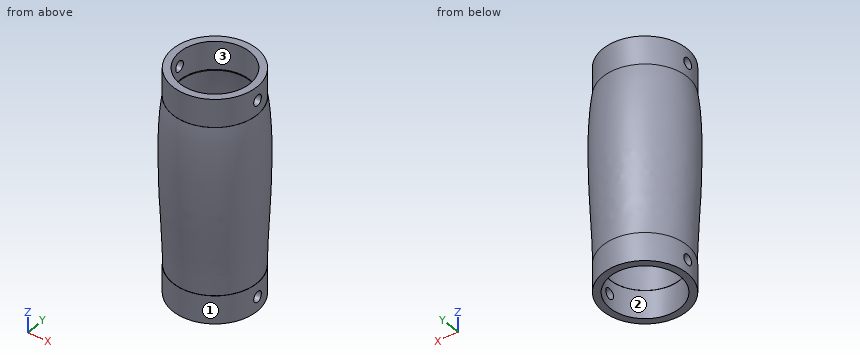
from build123d import *

# Parameters (mm, degrees)
F0_R          = 38.1
F0_R_2        = 31.75
F1_DEPTH      = 25.4
F5_R          = 38.1
F5_R_2        = 31.75
F6_DEPTH      = 25.4
F7_R          = 4.7625
F8_DEPTH      = 41.3056266711
F8_DEPTH_BACK = 41.3056266711


with BuildPart() as f1:
    # F0 (on Top) → F1 (new body)
    with BuildSketch(Plane.XY):
        Circle(F0_R)
        Circle(F0_R_2, mode=Mode.SUBTRACT)
    extrude(amount=F1_DEPTH)

    # F2 (on Front) → F3 (revolve)
    with BuildSketch(Plane.XZ):
        with BuildLine():
            add(Edge.make_bspline(
                [(-37.9096439485, 25.4), (-37.9096439485, 61.3283317127), (-45.343901962, 132.9952478409), (-38.2101392492, 177.8)],
                knots=[0, 0, 0, 0, 152.4002962511, 152.4002962511, 152.4002962511, 152.4002962511], degree=3))
            Line((-37.9096439485, 25.4), (-31.5596439485, 25.4))
            add(Edge.make_bspline(
                [(-31.5596439485, 25.4), (-31.5596439485, 30.0005361538), (-31.7962708065, 40.229659673), (-32.5871723352, 58.0663276532), (-33.5556486353, 77.7063467951), (-34.4446785922, 98.4319215024), (-34.9986327696, 119.5084440497), (-34.9638253583, 140.1883641654), (-34.0922055878, 159.7067304565), (-32.7967181283, 171.41530853), (-31.9391288783, 176.8015367165)],
                knots=[0, 0, 0, 0, 0.125, 0.25, 0.375, 0.5, 0.625, 0.75, 0.875, 1, 1, 1, 1], degree=3))
            Line((-31.9391288783, 176.8015367165), (-31.6526181996, 177.8))
            Line((-31.6526181996, 177.8), (-38.2101392492, 177.8))
        make_face()
    revolve(axis=Axis((0, 0, 43.0460348713), (0, 0, 1)))

    # F5 (on offset) → F6 (join)
    with BuildSketch(Plane.XY.offset(177.8)):
        Circle(F5_R)
        Circle(F5_R_2, mode=Mode.SUBTRACT)
    extrude(amount=F6_DEPTH)

    # F7 (on Right) → F8 (cut, two sides)
    with BuildSketch(Plane.YZ) as f8_sk:
        with Locations((0, 190.5)):
            Circle(F7_R)
        with Locations((0, 12.7)):
            Circle(F7_R)
    extrude(amount=-F8_DEPTH, mode=Mode.SUBTRACT)
    extrude(f8_sk.sketch, amount=F8_DEPTH_BACK, mode=Mode.SUBTRACT)


solid = f1.part
Input: part model. Units: mm. Frame: model coordinates. Face numbers are marked on the shaded views. Round coordinates to 2 decimals unless told otherwise and drop trailing zeros. Loops run counter-clockwise (first coordinate to the right, second up) from the corner with the lowest first, then second, coordinate; pieces in that order, holes last. Notation, with made-up numbers: M 82,-7.5 L 103,-7.5 A12 cw 103,2.5 Z; hole C -10.75,66 d9. An arc over 180 degrees is marked long. Answer as CSV lines item,"result". Start each with the question number.
(1) Draft query along Y for the marked faces 1, 2 and 3. Return one class per face: released by +Y, released by -Y, zero draft, split by the parting line, or undercut.
(2) Line query: line 1 (Y direction, x = 0, z = 183.75); line 2 (Y direction, x = -29, z = 128); line 3 (X direction, y = -5, z = 32). Output: solid intervals per line, ascending. Write a range as [from, to].
(3) Section B-B, the plane y = 0. State how many separate pieces and enclosed holes the cut face has, plus the area to 3 significant figures.
(4) First-contact query: pin 1 (12.5 mm diameter, centred on y = 0, z = 190.5, fed in from -X); pin 2 (3 mm diameter, centred on x = 12, z = 32, fed in from +Y); pin 3 (6 mm diameter, centred on y = 5.5, z = 80, fed in from -X); pin 4 (3 mm diameter, centred on x = 12.5, y = 29.5, fed in from -Z). Flat tips, straight axial feed; report the tip coordinate or a pass-through.
(5) Section A-A, the plane z = 12.7. Output: boundary loops of the cut face in (x, y), plus the area to 3 significant figures.
Values found:
1,face 1,"split by the parting line"
1,face 2,"undercut"
1,face 3,"undercut"
2,line 1,"y = [-38.1, -31.75], [31.75, 38.1]"
2,line 2,"y = [-29.41, -19.51], [19.51, 29.41]"
2,line 3,"x = [-37.65, -31.23], [31.23, 37.65]"
3,separate pieces,"6"
3,enclosed holes,"0"
3,area,"2,340 mm²"
4,pin 1,"stops at x = -38.1"
4,pin 2,"stops at y = 36.5"
4,pin 3,"stops at x = -39.96"
4,pin 4,"stops at z = 0"
5,outline,"M -37.8,-4.76 A38.1 ccw 37.8,-4.76 L 31.39,-4.76 A31.75 cw -31.39,-4.76 Z; M -37.8,4.76 L -31.39,4.76 A31.75 cw 31.39,4.76 L 37.8,4.76 A38.1 ccw Z"
5,area,"1,270 mm²"
